Study the drawing (mm; zero at the part's minimum x, y, z) and answer. A direction names the side the tool comes from. Give positions to 0.01 mm unless a question says otherwise; leave off trailing zeros. Write each loop counter-clockwise with the first axis right and the second up, starting at its lowest first coordinate (ties: lowest second). Pieces come first, ordered by that corner, then holes.
1) Find section A-A (x = 11). Determine the outline of the cut face in (y, z), plus the area to 3 significant figures.
2) Find section B-B (z = 3.5). Determine the outline of the cut face in (x, y).
3) A tool of negligible diameter and unlimited length cuts with its end or side. For the marked faces 1 and 2, from which of +Z, -Z, +X, -X, +Y, -Y can it reach the whole face along a straight path? Write none if from no direction.
4) Straight lines are drawn through the part: probe 1 along Z at (x, y) = (3.5, 5.75); probe 2 along X at (y, z) = (6, 4); probe 3 along Z at (x, y) = (2.75, 7). For each, find the intervals that lie inside material, in ascending order.
5) Given pin 1 Ø1 at (y, z) = (9.5, 4) entering from -X, flat-ended and moving along its own axis, determine where the tip first touches the part or whether it passes through.
6) Determine the mould class of the marked faces 3, 4 and 5 for opening direction X: pulls with the +X half, pulls with the -X half, needs draft (parallel to the pull), parting line crosses it, or undercut.
7) Find section D-D (y = 6.75). Determine the outline of the cut face in (x, z), plus the area to 3 significant figures.
8) Find section C-C (y = 9.5). Determine the outline of the cut face in (x, z), plus the area to 3 significant figures.
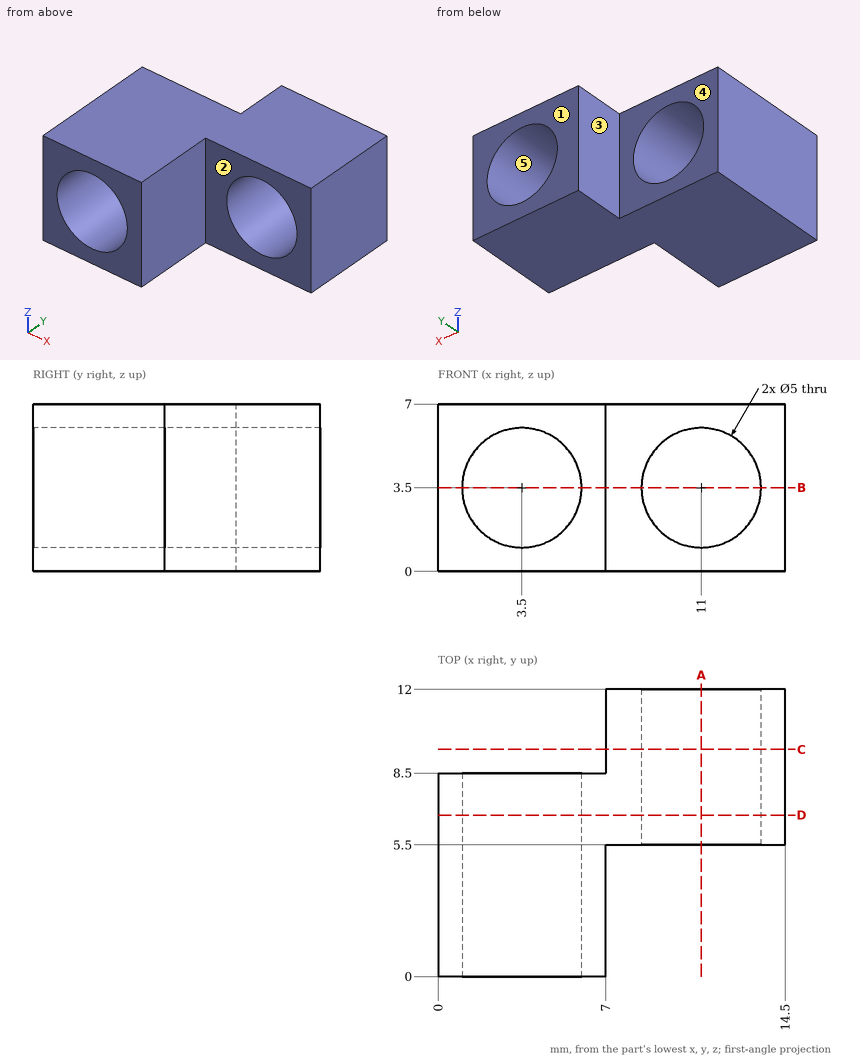
Results:
1. outline: (5.5, 0) - (12, 0) - (12, 1) - (5.5, 1) - close; (5.5, 6) - (12, 6) - (12, 7) - (5.5, 7) - close
1. area: 13.0 mm2
2. outline: (0, 0) - (1, 0) - (1, 8.5) - (0, 8.5) - close; (6, 0) - (7, 0) - (7, 5.5) - (8.5, 5.5) - (8.5, 12) - (7, 12) - (7, 8.5) - (6, 8.5) - close; (13.5, 5.5) - (14.5, 5.5) - (14.5, 12) - (13.5, 12) - close
3. face 1: +Z, -Z, +X, -X, +Y
3. face 2: +Z, -Z, +X, -Y
4. probe 1: z = 0 to 1, 6 to 7
4. probe 2: x = 0 to 1.05, 5.95 to 8.55, 13.45 to 14.5
4. probe 3: z = 0 to 1.12, 5.88 to 7
5. pin 1: stops at x = 7
6. face 3: pulls with the -X half
6. face 4: needs draft
6. face 5: undercut
7. outline: (0, 0) - (14.5, 0) - (14.5, 7) - (0, 7) - close; hole circle Ø5 at (3.5, 3.5); hole circle Ø5 at (11, 3.5)
7. area: 62.2 mm2
8. outline: (7, 0) - (14.5, 0) - (14.5, 7) - (7, 7) - close; hole circle Ø5 at (11, 3.5)
8. area: 32.9 mm2
